Check sheet for the drawn part. Datum: minimum x, y, z corner. Units: mm. A direction names the side the tool comes from. Coordinates: 2 decimals unless noted, no trailing zeros. Order: outer loops, then holes, each group sorted by start corner. A loop starts at its lowest first (then second) coordinate and runs counter-clockwise, first axis right, second up.
1. Cross-section at A-A (x = 9). Enter the section's corners in (y, z).
2. Thickness scan on line 1 (X direction, y = 7, z = 9); line 2 (Y direction, x = 3.5, z = 13.5); line 3 (Z direction, x = 5, y = 16.25). Record the ranges inside material, lowest first.
3. Cross-section at C-C (z = 7.5). Enter the section's corners in (x, y).
4. Set-up check for the marked faces 5, 6 and 7: record each of +Z, -Z, +X, -X, +Y, -Y from which the full face is reachable in a straight line by a thin tool's end or side.
5. Gauge pin test, flat ends, axial feed: pin 1 Ø1.6 at (x, y) = (5.5, 9) entering from -Z; pin 2 Ø2 at (x, y) = (3, 17.5) entering from +Z; pin 3 Ø0.6 at (x, y) = (6, 9.5) entering from +Z; pin 4 Ø1.2 at (y, z) = (2, 12.83) entering from -X. Record the tip position at first contact, or that the pin passes through.
6. Draft check along Y on the marked faces 1, 2, 3 and 4. Enter one of: released by +Y, released by -Y, zero draft, split by the parting line, or undercut.
7. Cross-section at B-B (y = 2). Enter the section's corners in (x, z), then the cut area to 3 significant figures.
8. Cross-section at D-D (x = 7). Enter the section's corners in (y, z), then the cut area to 3 significant figures.
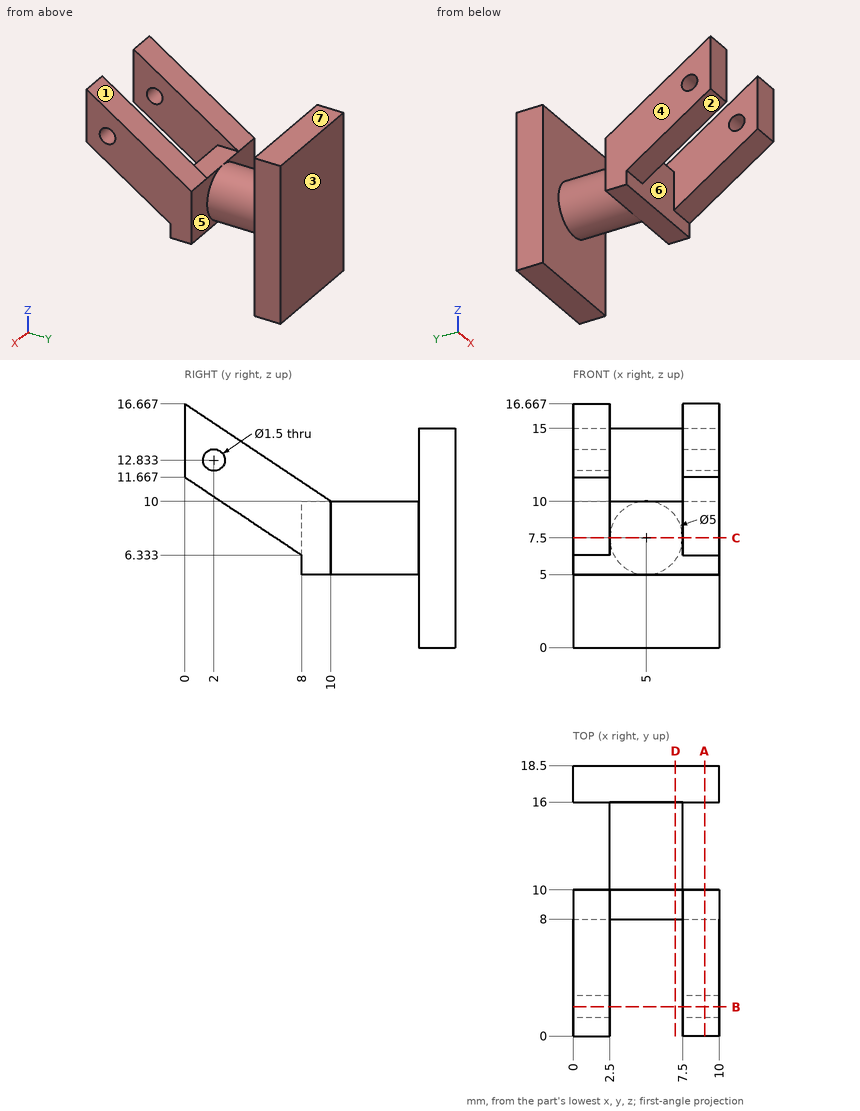
Data:
1. outline: (0, 11.67) - (8, 6.33) - (8, 5) - (10, 5) - (10, 10) - (0, 16.67) - close; (16, 0) - (18.5, 0) - (18.5, 15) - (16, 15) - close; hole circle Ø1.5 at (2, 12.83)
2. line 1: x = 0 to 2.5, 7.5 to 10
2. line 2: y = 16 to 18.5
2. line 3: z = 0 to 15
3. outline: (0, 6.25) - (2.5, 6.25) - (2.5, 8) - (7.5, 8) - (7.5, 6.25) - (10, 6.25) - (10, 10) - (7.5, 10) - (7.5, 16) - (10, 16) - (10, 18.5) - (0, 18.5) - (0, 16) - (2.5, 16) - (2.5, 10) - (0, 10) - close
4. face 5: +X
4. face 6: -Z, -Y
4. face 7: +Z, +X, -X, +Y
5. pin 1: stops at z = 5
5. pin 2: stops at z = 15
5. pin 3: stops at z = 10
5. pin 4: passes through
6. face 1: undercut
6. face 2: released by -Y
6. face 3: released by +Y
6. face 4: zero draft
7. outline: (0, 10.33) - (2.5, 10.33) - (2.5, 12.08) - (0, 12.08) - close; (0, 13.58) - (2.5, 13.58) - (2.5, 15.33) - (0, 15.33) - close; (7.5, 10.33) - (10, 10.33) - (10, 12.08) - (7.5, 12.08) - close; (7.5, 13.58) - (10, 13.58) - (10, 15.33) - (7.5, 15.33) - close
7. area: 17.5 mm2
8. outline: (8, 5) - (10, 5) - (10, 6) - (16, 6) - (16, 0) - (18.5, 0) - (18.5, 15) - (16, 15) - (16, 9) - (10, 9) - (10, 10) - (8, 10) - close
8. area: 65.5 mm2
